Solid Edge part; units mm, degrees
sketch "Sketch1" plane through (0, 0, 0) normal (0, 0, 1) x (1, 0, 0)
  line L0 (0, 0) -> (0, 50)
  arc A0 (0, -50) -> (0, 50) centre (0, 0) ccw
  line L1 (0, 0) -> (0, -50)
extrude "Protrusion1" add sketch "Sketch1" against normal blind 25
sketch "Sketch2" plane through (25, 0, 0) normal (0, 0, 1) x (0, 1, 0)
  line L0 (-15, -7) -> (-15, -25)
  line L1 (-15, -25) -> (15, -25)
  line L2 (15, -7) -> (15, -25)
  line L3 (0, -7) -> (15, -7)
  line L4 (0, -7) -> (-15, -7)
extrude "ExtrudedCutout_1" cut sketch "Sketch2" against normal blind 5
sketch "Sketch3" plane through (0, 0, 0) normal (0, -1, 0) x (1, 0, 0)
  line L0 (-18, 45) -> (-48, 45)
  line L1 (22, 5) -> (22, -25)
  arc A0 (22, -25) -> (-48, 45) centre (22, 45) cw
  arc A1 (22, 5) -> (-18, 45) centre (22, 45) cw
extrude "ExtrudedProtrusion_3" add sketch "Sketch3" along normal mid plane 30
sketch "Sketch4" plane through (-33, 0, 45) normal (0, 0, 1) x (0, 1, 0)
  line L0 (5, -30) -> (5, 30)
  line L1 (5, 30) -> (-5, 30)
  line L2 (-5, 30) -> (-5, -30)
  line L3 (-5, -30) -> (5, -30)
extrude "ExtrudedCutout_2" cut sketch "Sketch4" along normal mid plane 25.6
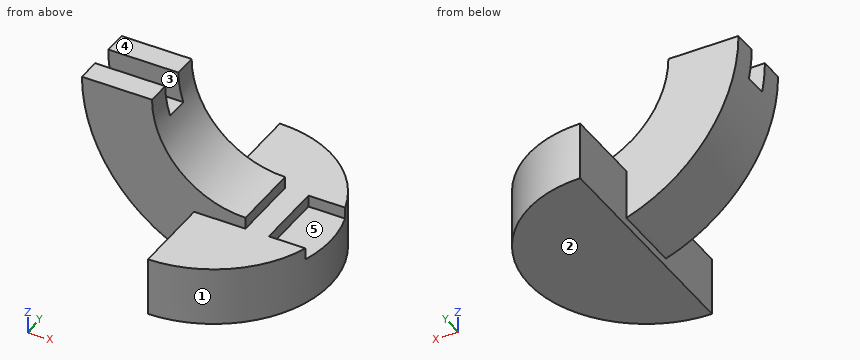
Read the model definition and answer for the solid it produces. Units are mm, in the model's axes. Face numbers are marked on the shaded views. A direction names the side the tool comes from. Round coordinates to 2 decimals unless told otherwise and drop trailing zeros. Write each loop counter-clockwise with the first axis right and the second up, starting at its lowest first coordinate (ties: lowest second). Pieces come first, ordered by that corner, then holes.
1. The part is cut by section C-C, the plane x = 35.5. Determine the outline of the cut face in (y, z), then the cut area to 3 significant figures.
2. The part is cut by section A-A, the plane y = 0. Determine the outline of the cut face in (x, z).
3. The part is cut by section B-B, the plane z = 33.5. Determine the outline of the cut face in (x, y), then the cut area to 3 significant figures.
4. The part is cut by section D-D, the plane z = -10. Determine the outline of the cut face in (x, y).
5. Straight lines are drawn through the part: L1, parallel to Y at x = -27.5, z = 42; L2, parallel to Y at x = -19, z = 31; L3, parallel to Z at x = 23.5, y = 26.5. For each, find the intervals that lie inside material, in ascending order.
6. Determine the mould class of the marked faces 1, 2 and 3 for opening direction Y: pulls with the +Y half, pulls with the -Y half, needs draft (parallel to the pull), parting line crosses it, or undercut.
7. Which of the six approach directions +Z, -Z, +X, -X, +Y, -Y give full straight-line access (tool end or side, diameter ignored) to the marked faces 4 and 5?
8. Given pin 1 Ø2 at (x, y) = (-22.5, 14) entering from -Z; pin 2 Ø12 at (y, z) = (-11.5, 25) entering from +X; pin 3 Ø10 at (x, z) = (-25.5, 37) entering from +Y; pin 4 Ø8 at (y, z) = (-22, 30.5) entering from +X, each flat-ended and moving along its own axis, determine where each tip first touches the part or whether it passes through.
Values:
1. outline: (-35.21, -25) - (35.21, -25) - (35.21, 0) - (15, 0) - (15, -5) - (-15, -5) - (-15, 0) - (-35.21, 0) - close
1. area: 1,610 mm2
2. outline: (-46.82, 32.2) arc R70 ccw to (0, -21.45) - (0, -25) - (50, -25) - (50, -5) - (32, -5) - (32, 0) - (22, 0) - (22, 5) arc R40 cw to (-15.9, 32.2) - close
3. outline: (-47.05, -15) - (-16.31, -15) - (-16.31, -5) - (-47.05, -5) - close; (-47.05, 5) - (-16.31, 5) - (-16.31, 15) - (-47.05, 15) - close
3. area: 615 mm2
4. outline: (-21.3, -15) - (0, -15) - (0, -50) arc R50 ccw to (0, 50) - (0, 15) - (-21.3, 15) - close
5. L1: y = -15 to -5, 5 to 15
5. L2: y = -15 to 15
5. L3: z = -25 to 0
6. face 1: parting line crosses it
6. face 2: needs draft
6. face 3: undercut
7. face 4: +Z, +X, -X, +Y, -Y
7. face 5: +Z, +X
8. pin 1: stops at z = -9.84
8. pin 2: stops at x = -8.4
8. pin 3: stops at y = 15
8. pin 4: passes through
